```python
from build123d import *

# Parameters (mm, degrees)
BOSS_EXTRUDE3_DEPTH = 3
BOSS_EXTRUDE4_DEPTH = 1.5


with BuildPart() as part:
    # Sketch1 → Boss-Extrude3 (new body)
    with BuildSketch(Plane.XY):
        with BuildLine():
            ThreePointArc((1.342685699, 34.173633039), (0.671472282, 34.193407624), (0, 34.2))
            Line((0, 34.2), (0, 4.5))
            Line((0, 4.5), (28, 4.5))
            Line((28, 4.5), (28, 1.5))
            Line((28, 1.5), (28, -12.5))
            Line((28, -12.5), (28, -17))
            Line((28, -17), (21.5, -23.5))
            Line((21.5, -23.5), (0, -23.5))
            Line((0, -23.5), (0, -36))
            ThreePointArc((0, -36), (35.993060657, -0.706812929), (1.413353367, 35.972245305))
            Line((1.413353367, 35.972245305), (1.342685699, 34.173633039))
        make_face()
        with BuildLine():
            Line((0, 4.5), (0, 34.2))
            ThreePointArc((0, 34.2), (-0.671472282, 34.193407624), (-1.342685699, 34.173633039))
            Line((-1.342685699, 34.173633039), (-1.413353367, 35.972245305))
            ThreePointArc((-1.413353367, 35.972245305), (-35.993060657, -0.706812929), (0, -36))
            Line((0, -36), (0, -23.5))
            Line((0, -23.5), (-21.5, -23.5))
            Line((-21.5, -23.5), (-28, -17))
            Line((-28, -17), (-28, 4.5))
            Line((-28, 4.5), (0, 4.5))
        make_face()
    extrude(amount=-BOSS_EXTRUDE3_DEPTH)

    # Sketch1_9 → Boss-Extrude4 (add)
    with BuildSketch(Plane.XY):
        Polygon((28, 4.5), (0, 4.5), (0, -23.5), (21.5, -23.5), (28, -17), (28, -12.5), (24.9, -12.5), (24.9, 1.5), (28, 1.5), align=None)
        Polygon((0, -23.5), (0, 4.5), (-28, 4.5), (-28, -17), (-21.5, -23.5), align=None)
    extrude(amount=-BOSS_EXTRUDE4_DEPTH)


solid = part.part
```
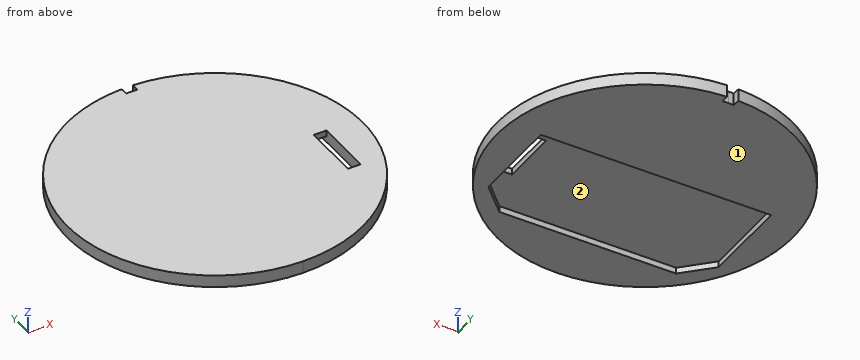
Design review of the part built by this model. Coordinates are the model's own, in mm. Face numbers are marked on the shaded views. Give positions to 0.01 mm unless a question says otherwise; leave off trailing zeros. Order: outer loops, then holes, each group sorted by start corner. A loop starts at its lowest first (then second) coordinate and runs counter-clockwise, first axis right, second up. Notation, with made-up numbers: M -11.5,-25 L 17.5,-25 A13 cw 17.5,-10 Z; hole C 86.25,-29 d3. An arc over 180 degrees is marked long. One line per question, with ' | ' between items. Start each with the question number.
Q1. We need section C-C (x = -8.5). Write out the cut boundary in (y, z), plus the area to 3 significant figures.
Q2. For L1, parallel to Y at x = 26, z = -0.95; L2, parallel to Y at x = 18, z = -2.4; L3, parallel to Z at x = 20.5, y = -1.5, list the stretches that pass through material, from the lowest coordinate up. Write a range as [from, to].
Q3. For pin 1 Ø1 at (y, z) = (-8.5, -1) entering from +X; pin 2 Ø1.2 at (x, z) = (27, -0.5) entering from -Y; pin 3 Ø1.6 at (y, z) = (-1.5, -2) entering from +X, all flat-tipped, find the tip position at first contact; note any pin that passes through.
Q4. The part is to be moulded in two halves that separate along X. For the marked faces 1 and 2, say which applies: +X half, -X half, draft (parallel to the pull), parting line (faces both ways), or undercut.
Q5. We need section A-A (y = 0). Write out the cut boundary in (x, z), plus the area to 3 significant figures.
Q6. We need section D-D (y = 20). Write out the cut boundary in (x, z).
Q7. We need section B-B (z = -2.3). Write out the cut boundary in (x, y), plus the area to 3 significant figures.
Returned:
1) outline: M -34.98,-3 L -23.5,-3 L -23.5,-1.5 L 4.5,-1.5 L 4.5,-3 L 34.98,-3 L 34.98,0 L -34.98,0 Z | area: 168 mm2
2) L1: [-24.9, -12.5], [1.5, 24.9] | L2: [-31.18, -23.5], [4.5, 31.18] | L3: [-1.5, 0]
3) pin 1: x = 35.1 | pin 2: y = -24.48 | pin 3: x = 35.99
4) face 1: draft | face 2: undercut
5) outline: M -36,-3 L -28,-3 L -28,-1.5 L 24.9,-1.5 L 24.9,0 L -36,0 Z; M 28,-3 L 36,-3 L 36,0 L 28,0 Z | area: 127 mm2
6) outline: M -29.93,-3 L 29.93,-3 L 29.93,0 L -29.93,0 Z
7) outline: M -1.41,35.97 A36 ccw long 1.41,35.97 L 1.34,34.17 A34.2 ccw -1.34,34.17 Z; hole M -28,-17 L -21.5,-23.5 L 21.5,-23.5 L 28,-17 L 28,4.5 L -28,4.5 Z | area: 2,540 mm2
